Print and shaded views of the part. All mm, measured from the part's lowest x, y and z. A direction names the side the tool comes from. Round coordinates to 2 decimals unless told otherwise and drop trailing zeros. Return JSON: item names as keys, results as strings. Group by question number.
Item 1: Drop flat-ended pins along their axis: pin 1 (2 mm diameter, centred on x = 21, z = 6.5, fed in from +Y); pin 2 (4 mm diameter, centred on x = 37, y = 19.14, fed in from -Z); pin 3 (6 mm diameter, centred on y = 13.5, z = 3.5, fed in from -X); pin 4 (5 mm diameter, centred on y = 12, z = 10.5, fed in from -X). Give the stop position or say it passes through.
Item 2: Probe probe 1 along X at (y, z) = (3.5, 7.5) (1 decimal); probe 2 along Y at (x, z) = (27, 10.75) (1 decimal); probe 3 along Y at (x, z) = (31, 12.5) (1 decimal). List the from-to ranges inside material, lowest first.
Item 3: Tool access for the marked faces 4 and 5: list every direction of +Z, -Z, +X, -X, +Y, -Y with a clear straight run to the whole face (end or side of a thin tool).
Item 4: Two-plate mould, pull along X, no slides. Class the marked faces 1, 2 and 3: released by +X, released by -X, zero draft, split by the parting line, or undercut.
Item 5: Saw through at A-A on z = 7.5. State how many separate pieces and enclosed holes the cut face has, and give its area (3 significant figures).
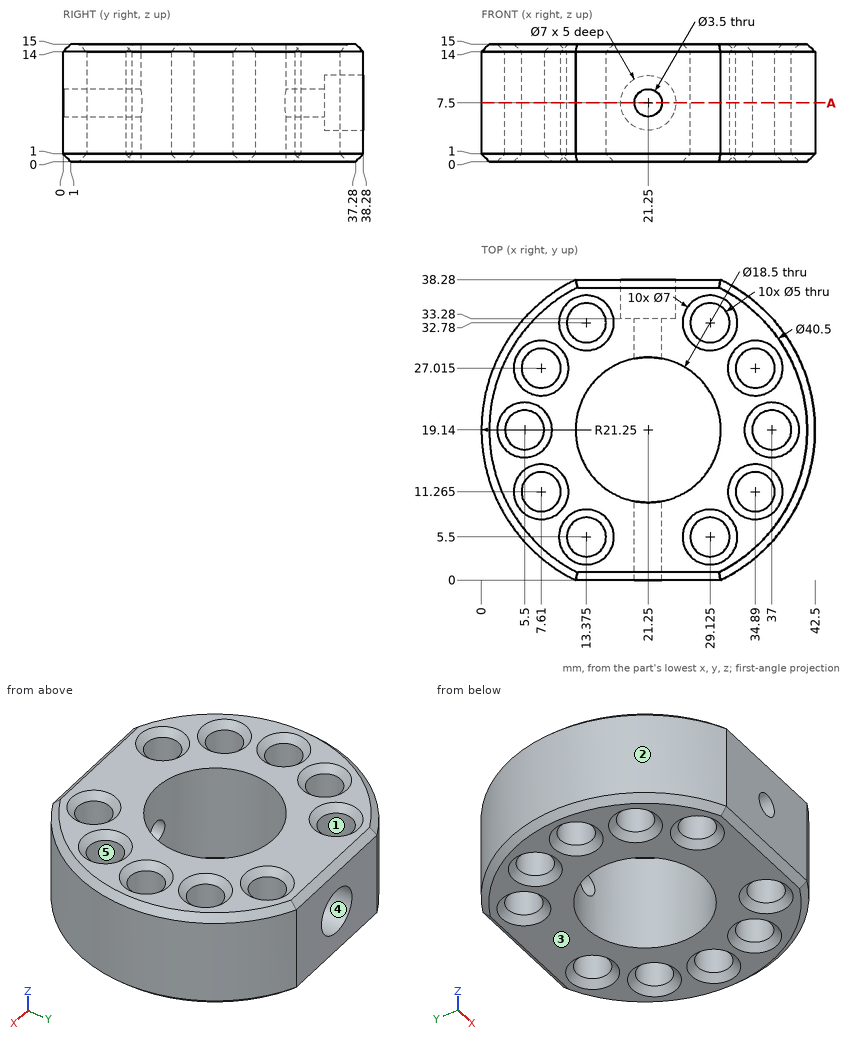
Filled in:
{
 "1": {"pin 1": "stops at y = 33.28", "pin 2": "passes through", "pin 3": "stops at x = 0.16", "pin 4": "stops at x = 0.51"},
 "2": {"probe 1": "x = 6.9 to 11.9, 14.9 to 19.5, 23 to 27.6, 30.6 to 35.6", "probe 2": "y = 0 to 4.2, 6.8 to 11.9, 26.4 to 31.5, 34.1 to 38.3", "probe 3": "y = 0.3 to 3.8, 7.2 to 31.1, 34.4 to 38"},
 "3": {"face 4": "+Y", "face 5": "+Z, -Z"},
 "4": {"face 1": "undercut", "face 2": "released by -X", "face 3": "zero draft"},
 "5": {"separate pieces": "2", "enclosed holes": "10", "area": "814 mm^2"}
}
